Autodesk Inventor part; units mm, degrees
ref_plane "YZ Plane" through (0, 0, 0) normal (1, 0, 0) x (0, 1, 0)
ref_plane "XZ Plane" through (0, 0, 0) normal (0, 1, 0) x (-1, 0, 0)
ref_plane "XY Plane" through (0, 0, 0) normal (0, 0, 1) x (1, 0, 0)
sketch "Sketch1" plane through (0, 0, 0) normal (0, 1, 0) x (-1, 0, 0)
  line L0 (0, -228) -> (-183, -228)
  line L1 (-183, -228) -> (-183, 0)
  line L2 (-183, 0) -> (0, 0)
  line L3 (0, 0) -> (0, -228)
  dimension "d26" = 228
  dimension "d27" = 183
extrude "base" add sketch "Sketch1" along normal blind 3
sketch "Sketch5" plane through (0, 3, 0) normal (0, 1, 0) x (1, 0, 0)
  line L0 (0, 228) -> (0, 0)
  line L1 (0, 0) -> (183, 0)
  line L2 (183, 0) -> (183, 228)
  line L3 (183, 228) -> (0, 228)
  point P0 (111.5, 114)
  dimension "d46" = 114
  dimension "d47" = 111.5
  dimension "d48" = 183
  dimension "d49" = 228
hole "centreHole" at (111.5, 3, -114) direction (0, -1, 0) diameter 17 end through all
chamfer "holeChamfer" distance 0.5 angle 45 2 edges at (111.5, 0, -122.5) (111.5, 3, -122.5)
sketch "Sketch7" plane through (0, 3, 0) normal (0, 1, 0) x (1, 0, 0)
  line L0 (183, 228) -> (0, 228)
  line L1 (0, 0) -> (183, 0)
  line L2 (183, 0) -> (183, 228)
  line L3 (183, 228) -> (0, 228)
  line L4 (0, 228) -> (0, 0)
  line L5 (3, 3) -> (180, 3)
  line L6 (180, 3) -> (180, 225)
  line L7 (180, 225) -> (3, 225)
  line L8 (3, 225) -> (3, 3)
  dimension "d29" = 3
extrude "walls" add sketch "Sketch7" along normal blind 115
sketch "Sketch10" plane through (180, 3, -225) normal (-1, 0, 0) x (0, 0, 1)
  line L0 (59, 48) -> (107, 48)
  line L1 (107, 48) -> (107, 42)
  line L2 (107, 42) -> (59, 42)
  line L3 (59, 42) -> (59, 48)
  line L4 (222, 0) -> (222, 115)
  line L5 (222, 0) -> (0, 0)
  line L6 (83, 48) -> (83, 42)
  point P0 (225, -3)
  dimension "d60" = 6
  dimension "d61" = 48
  dimension "d91" = 139
  dimension "d92" = 222
  dimension "d118" = 48
extrude "platform" add sketch "Sketch10" along normal blind 90
sketch "Sketch11" plane through (180, 51, -118) normal (0, 1, 0) x (1, 0, 0)
  circle A0 centre (-68.5, 24) radius 18
  line L0 (-68.5, 24) -> (-50.5, 24)
  line L1 (-68.5, 24) -> (-77.5, 8.4115)
  line L2 (-68.5, 24) -> (-77.5, 39.5885)
  line L3 (0, 0) -> (-90, 0)
  line L4 (0, 48) -> (-90, 48)
  circle A1 centre (-68.5, -4) radius 9
  line L5 (-68.5, -4) -> (-68.5, 60.8189)
  point P0 (-180, -118)
  dimension "d68" = 36
  dimension "d69" = 120
  dimension "d70" = 120
  dimension "d74" = 48
  dimension "d82" = 28
hole "motorScrewHoles" at (102.5, 51, -157.5885) at (129.5, 51, -142) at (102.5, 51, -126.4115) direction (0, -1, 0) diameter 6 depth 6
sketch "Sketch12" plane through (180, 51, -118) normal (0, 1, 0) x (1, 0, 0)
  circle A0 centre (-68.5, -4) radius 9
  line L0 (-68.5, -4) -> (-68.5, 71.2028)
  circle A1 centre (-68.5, 24.4211) radius 12.5
  point P0 (-180, -118)
  dimension "d83" = 25
extrude "motorShaftHole" cut sketch "Sketch12" against normal up to surface (6 mm away) contours A1 L0 | L0 A1
chamfer "Chamfer2" distance 0.5 angle 45 2 edges at (99, 45, -142.4211) (99, 51, -142.4211)
sketch "Sketch13" plane through (3, 3, -225) normal (0, 0, 1) x (1, 0, 0)
  line L0 (177, 0) -> (0, 0)
  line L1 (64, 0) -> (67, 0)
  line L2 (67, 0) -> (67, 65)
  line L3 (67, 65) -> (64, 65)
  line L4 (64, 65) -> (64, 0)
  line L5 (87, 42) -> (87, 48)
  point P0 (-3, -3)
  dimension "d93" = 3
  dimension "d94" = 65
  dimension "d95" = 20
extrude "Extrusion8" add sketch "Sketch13" along normal blind 54
sketch "Sketch14" plane through (67, 3, -225) normal (-1, 0, 0) x (0, 0, 1)
  circle A0 centre (27, 36) radius 18
  line L0 (27, 36) -> (11.4115, 27)
  line L1 (27, 36) -> (27, 54)
  line L2 (27, 36) -> (42.5885, 27)
  line L3 (54, 0) -> (0, 0)
  line L4 (54, 65) -> (54, 0)
  line L5 (0, 0) -> (0, 115)
  point P0 (225, -3)
  dimension "d98" = 36
  dimension "d99" = 120
  dimension "d100" = 120
  dimension "d101" = 36
  dimension "d114" = 27
hole "Hole4" at (67, 30, -213.5885) at (67, 57, -198) at (67, 30, -182.4115) direction (1, 0, 0) diameter 6 depth 3
fillet "Fillet2" radius 1 10 edges at (180, 51, -142) (180, 45, -142) (180, 48, -118) (180, 48, -166) (68.5, 68, -225) (67, 35.5, -225) (70, 35.5, -225) (70, 3, -198) (67, 3, -198) (68.5, 3, -171)
sketch "Sketch15" plane through (67, 4, -171) normal (-1, 0, 0) x (0, 0, 1)
  circle A0 centre (-27, 36) radius 12.5
  line L0 (0, 0) -> (-53, 0)
  line L1 (-54, 65) -> (-54, -1)
  point P0 (171, -4)
  dimension "d111" = 25
  dimension "d115" = 36
  dimension "d116" = 27
extrude "Extrusion9" cut sketch "Sketch15" against normal up to surface (3 mm away)
fillet "Fillet3" radius 30 1 edges at (68.5, 68, -171)
sketch "Sketch16" plane through (0, 3, 0) normal (0, 1, 0) x (1, 0, 0)
  circle A0 centre (95, 176) radius 10
  line L0 (67, 171) -> (70, 171)
  line L1 (70, 201) -> (70, 171)
  point P0 (0, 0)
  dimension "d119" = 20
  dimension "d121" = 25
  dimension "d127" = 5
extrude "Extrusion10" cut sketch "Sketch16" against normal blind 50
chamfer "Chamfer3" distance 0.5 angle 45 2 edges at (85, 3, -176) (85, 0, -176)
sketch "Sketch17" plane through (0, 118, 0) normal (0, 1, 0) x (1, 0, 0)
  line L0 (0, 228) -> (183, 228)
  line L1 (183, 228) -> (183, 0)
  line L2 (183, 0) -> (0, 0)
  line L3 (0, 0) -> (0, 228)
  point P0 (0, 0)
extrude "Extrusion11" add sketch "Sketch17" along normal blind 3
chamfer "Chamfer4" distance 1.5 angle 45 11 edges at (0, 60.5, -228) (0, 121, -114) (91.5, 121, -228) (183, 121, -114) (183, 60.5, -228) (91.5, 121, 0) (0, 60.5, 0) (0, 0, -114) (91.5, 0, -228) (91.5, 0, 0) (183, 0, -114)
sketch "Sketch18" plane through (0, 121, 0) normal (0, 1, 0) x (1, 0, 0)
  circle A0 centre (61, 152) radius 27.5
  line L0 (183, 0) -> (183, 226.5)
  line L1 (0, 226.5) -> (0, 1.5)
  line L2 (181.5, 228) -> (1.5, 228)
  line L3 (1.5, 0) -> (183, 0)
  line L4 (61, 152) -> (86.8415, 142.5944)
  line L5 (61, 152) -> (39.9338, 134.3233)
  line L6 (61, 152) -> (56.2247, 179.0822)
  line L7 (61, 152) -> (33.5, 152)
  point P0 (0, 0)
  dimension "d133" = 55
  dimension "d134" = 183
  dimension "d135" = 61
  dimension "d136" = 228
  dimension "d137" = 76
  dimension "d138" = 120
  dimension "d147" = 120
  dimension "d149" = 80
hole "Hole5" at (56.2247, 121, -179.0822) at (86.8415, 121, -142.5944) at (39.9338, 121, -134.3233) direction (0, -1, 0) diameter 8 depth 3
equation "\"d0\" = t"
equation "\"d29\" = t"
equation "\"d91\" = 0.5 * d92 + pd"
equation "\"d68\" = d72"
equation "\"d82\" = pd"
equation "\"d93\" = t"
equation "\"d128\" = t"
equation "\"d135\" = 0.333333 * d134"
equation "\"d137\" = 0.333333 * d136"
equation "\"t\" = 3"
equation "\"pd\" = 28"
equation "\"dmotorpattern\" = 36"
equation "\"d72\" = 36"
equation "\"d73\" = 28"
properties part number "box" material "Aluminum 6061"
Read the model definition and answer for the solid it produces. Units are mm, in the model's axes. A direction names the side the tool comes from. Round coordinates to 2 decimals unless told otherwise and drop trailing zeros. Write each loop counter-clockwise with the first axis right and the second up, starting at its lowest first coordinate (ties: lowest second). Pieces come first, ordered by that corner, then holes. Notation, with made-up numbers: (-12, 33.25) - (-6, 33.25) arc R18 cw to (-6, 39.25) - close; hole circle Ø6 at (80.25, 45). An arc over 180 degrees is marked (long way). Use a Markdown table: item, result.
(1) The part is cut by section A-A (x = 129.5). Write down the section's boundary in (y, z), then the cut area to 3 significant figures.
Reported:
| item | result |
|---|---|
| outline | (0, -226.5) - (1.5, -228) - (119.5, -228) - (121, -226.5) - (121, -1.5) - (119.5, 0) - (1.5, 0) - (0, -1.5) - close; (45, -166) - (51, -166) - (51, -145) - (45, -145) - close; (45, -139) - (51, -139) - (51, -118) - (45, -118) - close; hole (3, -225) - (118, -225) - (118, -3) - (3, -3) - close |
| area | 2,310 mm2 |
(2) The part is cut by section B-B (y = 96.5). Write down the section's boundary in (x, z), then the cut area to 3 significant figures.
Reported:
| item | result |
|---|---|
| outline | (0, -226.5) - (1.5, -228) - (181.5, -228) - (183, -226.5) - (183, 0) - (1.5, 0) - (0, -1.5) - close; hole (3, -225) - (180, -225) - (180, -3) - (3, -3) - close |
| area | 2,430 mm2 |
(3) The part is cut by section D-D (z = -114). Write down the section's boundary in (x, y).
Reported:
| item | result |
|---|---|
| outline | (0, 1.5) - (1.5, 0) - (102.5, 0) - (103, 0.5) - (103, 2.5) - (102.5, 3) - (3, 3) - (3, 118) - (180, 118) - (180, 3) - (120.5, 3) - (120, 2.5) - (120, 0.5) - (120.5, 0) - (181.5, 0) - (183, 1.5) - (183, 119.5) - (181.5, 121) - (1.5, 121) - (0, 119.5) - close |
(4) The part is cut by section C-C (x = 95). Write down the section's boundary in (y, z), then the cut area to 3 significant figures.
Reported:
| item | result |
|---|---|
| outline | (0, -226.5) - (1.5, -228) - (119.5, -228) - (121, -226.5) - (121, -1.5) - (119.5, 0) - (1.5, 0) - (0, -1.5) - (0, -165.5) - (0.5, -166) - (2.5, -166) - (3, -165.5) - (3, -3) - (118, -3) - (118, -225) - (3, -225) - (3, -186.5) - (2.5, -186) - (0.5, -186) - (0, -186.5) - close; (45, -166) - (51, -166) - (51, -118) - (45, -118) - close |
| area | 2,280 mm2 |
(5) Each of these flat-tipped pins is pushed along its axis until it touches: pin 1 Ø16 at (x, z) = (95, -176) entering from -Y; pin 2 Ø7 at (x, z) = (56.22, -179.08) entering from +Y. Where does it stop, or does it pass through?
Reported:
| item | result |
|---|---|
| pin 1 | y = 118 |
| pin 2 | y = 3 |
(6) The mould has two halves that part along X. Classify faces 1 (the flat face through (183, 60, -115)), 2 (the flat face through (90, 118, -116)): released by +X, released by -X, zero draft, split by the parting line, or undercut.
Reported:
| item | result |
|---|---|
| face 1 | released by +X |
| face 2 | undercut |
(7) Which of the six approach directions +Z, -Z, +X, -X, +Y, -Y give full straight-line access (tool end or side, diameter ignored) to faces 3 (the flat face through (135, 48, -118)), 4 (the cylindrical face through (56.05, 119.48, -183.08)), 5 (the cylindrical face through (92.83, 1.51, -166.24))?
Reported:
| item | result |
|---|---|
| face 3 | none |
| face 4 | +Y |
| face 5 | -Y |
(8) Straight lines are drawn through the part: line 1 along Z through (x, y) = (111, 49); line 2 along Y through (x, z) = (138, -130.5); line 3 along Y through (x, z) = (12, -140). For each, find the intervals that lie inside material, in ascending order. Write a range as [from, to].
Reported:
| item | result |
|---|---|
| line 1 | [-228, -225], [-166, -154.91], [-129.93, -118], [-3, 0] |
| line 2 | [0, 3], [45, 51], [118, 121] |
| line 3 | [0, 3], [118, 121] |
